```python
from build123d import *

# Parameters (mm, degrees)
BOSS_EXTRUDE1_DEPTH = 12.7
SKETCH2_R           = 9.525
CUT_EXTRUDE1_DEPTH  = 12.7
SKETCH3_R           = 6.5484375
CUT_EXTRUDE2_DEPTH  = 68.319185137
FILLET3_START       = -1
FILLET3_DEPTH       = 26.4
CUT_EXTRUDE3_DEPTH  = 68.319185137
FILLET4_R           = 5.08


with BuildPart() as part:
    # Sketch1 → Boss-Extrude1 (new, symmetric)
    with BuildSketch(Plane.XY):
        Polygon((0, 0), (63.3062413, 0), (63.3062413, 16.117198375), (32.943565298, 25.4), (32.943565298, 6.35), (0, 6.35), align=None)
    extrude(amount=BOSS_EXTRUDE1_DEPTH, both=True)

    # Sketch2 → Cut-Extrude1 (cut)
    with BuildSketch(Plane(origin=(9.91780582, 32.439681136, 0), x_dir=(0.9563047559630374, -0.29237170472273033, 0), z_dir=(0.29237170472273033, 0.9563047559630374, 0))):
        with Locations(Location((39.952846873, 0, 0), (0, 0, 180))):
            Circle(SKETCH2_R)
    extrude(amount=-CUT_EXTRUDE1_DEPTH, mode=Mode.SUBTRACT)

    # Sketch3 → Cut-Extrude2 (cut, through all)
    with BuildSketch(Plane(origin=(0, 6.35, 0), x_dir=(1, 0, 0), z_dir=(0, 1, 0))):
        with Locations(Location((16.471782649, 0, 0), (0, 0, 180))):
            Circle(SKETCH3_R)
    extrude(amount=-CUT_EXTRUDE2_DEPTH, mode=Mode.SUBTRACT)

    # Fillet3: read off the stored shape, not the designer's step
    # Fillet3 outline → Fillet3 (cut)
    with BuildSketch(Plane(origin=(0, 0, 0), x_dir=(1, 0, 0), z_dir=(0, 1, 0)).offset(FILLET3_START)):
        with BuildLine():
            ThreePointArc((50.6062413, 12.7), (59.586497421, 8.980256121), (63.3062413, 0))
            Line((63.3062413, 0), (63.3062413, 12.7))
            Line((63.3062413, 12.7), (50.6062413, 12.7))
        make_face()
        with BuildLine():
            ThreePointArc((63.3062413, 0), (59.586497421, -8.980256121), (50.6062413, -12.7))
            Line((50.6062413, -12.7), (63.3062413, -12.7))
            Line((63.3062413, -12.7), (63.3062413, 0))
        make_face()
    extrude(amount=FILLET3_DEPTH, mode=Mode.SUBTRACT)

    # Sketch4 → Cut-Extrude3 (cut, through all)
    with BuildSketch(Plane(origin=(0, 6.35, 0), x_dir=(1, 0, 0), z_dir=(0, 1, 0))):
        with BuildLine():
            Line((16.471782649, 12.7), (0, 12.7))
            Line((0, 12.7), (0, -12.7))
            Line((0, -12.7), (16.471782649, -12.7))
            ThreePointArc((16.471782649, -12.7), (3.771782649, 0), (16.471782649, 12.7))
        make_face()
    extrude(amount=-CUT_EXTRUDE3_DEPTH, mode=Mode.SUBTRACT)

    # Fillet4
    fillet4_edges = [part.edges().sort_by_distance(p)[0] for p in [
        (32.943565298, 6.35, 0),
    ]]
    fillet(fillet4_edges, radius=FILLET4_R)


solid = part.part
```
Input: part model. Units: mm. Frame: model coordinates. A direction names the side the tool comes from. Give positions to 0.01 mm unless a question says otherwise; leave off trailing zeros. Order: outer loops, then holes, each group sorted by start corner. A loop starts at its lowest first (then second) coordinate and runs counter-clockwise, first axis right, second up. Notation, with made-up numbers: (-12.5, -1) - (11.5, -1) arc R21 cw to (11.5, 27) - close; hole circle Ø10 at (39, -31.5). An arc over 180 degrees is marked (long way). One line per item, written item: value.
1. Cut plane A-A, the plane z = -3.5. Output: boundary loops of the cut face in (x, y).
Determined:
outline: (4.26, 0) - (10.94, 0) - (10.94, 6.35) - (4.26, 6.35) - close; (22.01, 0) - (62.81, 0) - (62.81, 16.27) - (56.6, 18.17) - (52.88, 6.02) - (35.94, 11.2) - (39.65, 23.35) - (32.94, 25.4) - (32.94, 11.43) arc R5.08 cw to (27.86, 6.35) - (22.01, 6.35) - close
2. Line query: probe 1 along Y at (x, z) = (23, -2.5); probe 2 along Z at (x, y) = (52.5, 9.25); probe 3 along Z at (x, y) = (55.5, 14.5). Output: solid intervals per line, ascending.
Determined:
probe 1: 0 to 6.35
probe 2: -12.56 to -5.81, 5.81 to 12.56
probe 3: -11.72 to -3.44, 3.44 to 11.72
3. Pin query (flat end, axial travel): pin 1 Ø12 at (x, z) = (10.5, -4.5) entering from +Y; pin 2 Ø12 at (y, z) = (14.5, -4) entering from -X; pin 3 Ø6 at (y, z) = (10.5, 10) entering from +X; pin 4 Ø12 at (y, z) = (17.5, -4) entering from +X. Return the tip coordinate at first contact, or that it passes through.
Determined:
pin 1: y = 6.35
pin 2: x = 32.01
pin 3: x = 61.2
pin 4: x = 63.31
4. Draft query along Z for faces 4 (the face through (37, 10, 12.7)), 5 (the face through (55.4, 12, 0.4)), 6 (the face through (13, 6.35, 6)). Return one class per face: released by +Z, released by -Z, zero draft, split by the parting line, or undercut.
Determined:
face 4: released by +Z
face 5: undercut
face 6: zero draft
5. Cut plane B-B, the plane x = 21.5. Output: boundary loops of the cut face in (y, z).
Determined:
outline: (0, -12.7) - (6.35, -12.7) - (6.35, -4.2) - (0, -4.2) - close; (0, 4.2) - (6.35, 4.2) - (6.35, 12.7) - (0, 12.7) - close
6. Cut plane D-D, the plane x = 31.5. Output: boundary loops of the cut face in (y, z).
Determined:
outline: (0, -12.7) - (7.88, -12.7) - (7.88, 12.7) - (0, 12.7) - close
7. Reachability of faces 1 (the face through (44.539, 8.575, 0.133)), 2 (the face through (33, 0, 0)), 3 (the face through (32.944, 19, 0)) from +Z, -Z, +X, -X, +Y, -Y: full face, straight path, thin tool, end or side. Return the list, or none.
Determined:
face 1: none
face 2: +Z, -Z, +X, -X, -Y
face 3: +Z, -Z, -X, +Y
8. Cut plane C-C, the plane z = 4.75. Output: boundary loops of the cut face in (x, y), and give its area (3 significant figures).
Determined:
outline: (4.69, 0) - (11.96, 0) - (11.96, 6.35) - (4.69, 6.35) - close; (20.98, 0) - (62.38, 0) - (62.38, 16.4) - (56.02, 18.34) - (52.31, 6.2) - (36.52, 11.03) - (40.23, 23.17) - (32.94, 25.4) - (32.94, 11.43) arc R5.08 cw to (27.86, 6.35) - (20.98, 6.35) - close
area: 533 mm2
